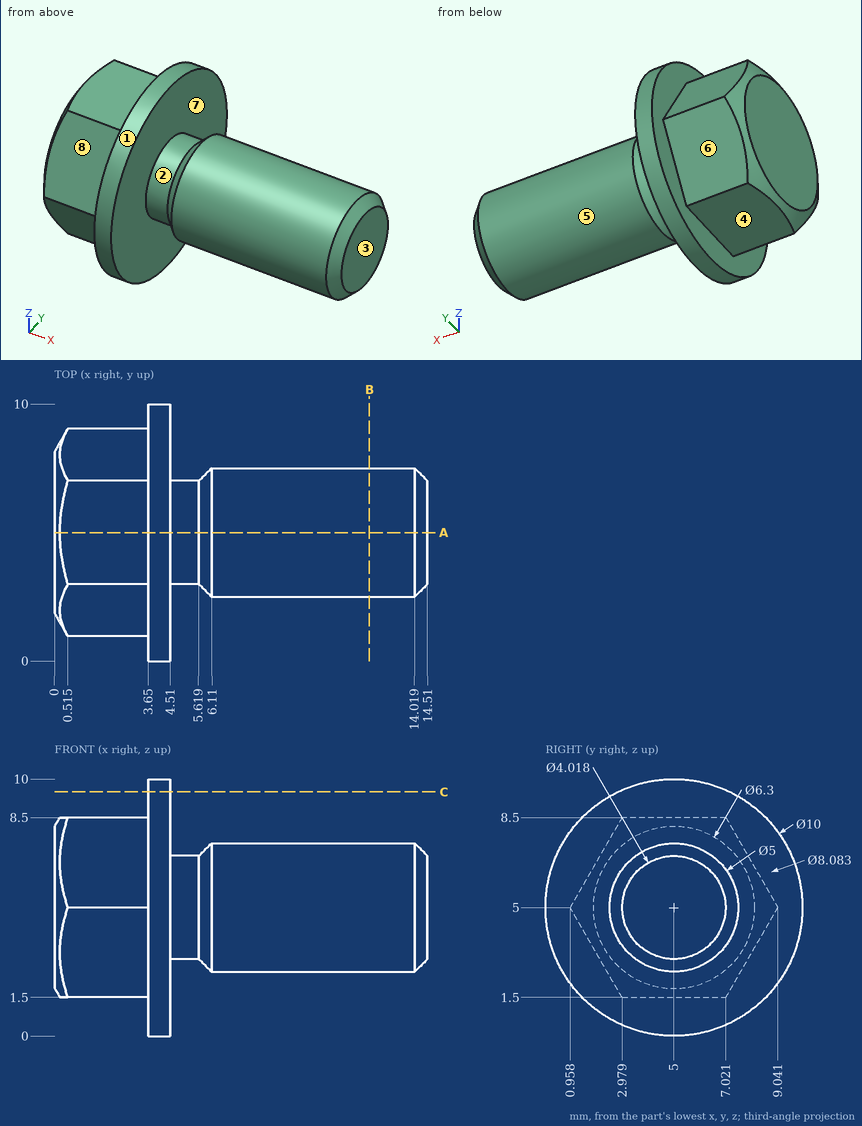
Here's the drawing with two shaded views (mm, measured from the low corner). I have some questions. A direction names the side the tool comes from. Give positions to 0.01 mm unless a question says otherwise; leave off trailing zeros. Loops run counter-clockwise (first coordinate to the right, second up) from the corner with the lowest first, then second, coordinate; pieces in that order, holes last. Notation, with made-up numbers: (-39, 73.5) -> (-6, 73.5) arc R29 ccw to (-6, 100.5) -> close; hole circle Ø10 at (64.5, 29.25). An arc over 180 degrees is marked (long way). Use one line per item in the form item = value.
1) For the marked faces 4, 5, 6, 7 and 8, which set-ups out of +Z, -Z, +X, -X, +Y, -Y let a thin tool reach every point of the face, with its end or its side?
Answers:
face_4 = -Z, -X, +Y, -Y
face_5 = +X
face_6 = -Z, -X, +Y
face_7 = none
face_8 = +Z, -X, -Y
2) We'd pull the mould along X, two halves only. Please class the marked faces 1, 2 and 3: released by +X, released by -X, zero draft, split by the parting line, or undercut.
Answers:
face_1 = zero draft
face_2 = undercut
face_3 = released by +X
3) I need wall thicknesses on line 1 along Z through (x, y) = (2, 4.25); line 2 along X through (y, z) = (2.5, 5.5); line 3 along X through (y, z) = (1.5, 3.25). Which ranges of each line are inside material? Lowest first, please.
Answers:
line_1 = 1.5 to 8.5
line_2 = 0 to 4.51
line_3 = 3.65 to 4.51
4) If we section it at B-B (x = 12.25): Please give me the cut outline in (y, z).
Answers:
outline = circle Ø5 at (5, 5)
5) If we section it at A-A (y = 5): Please give me the cut outline in (x, z).
Answers:
outline = (0, 1.85) -> (0.2, 1.5) -> (3.65, 1.5) -> (3.65, 0) -> (4.51, 0) -> (4.51, 2.99) -> (5.62, 2.99) -> (6.11, 2.5) -> (14.02, 2.5) -> (14.51, 2.99) -> (14.51, 7.01) -> (14.02, 7.5) -> (6.11, 7.5) -> (5.62, 7.01) -> (4.51, 7.01) -> (4.51, 10) -> (3.65, 10) -> (3.65, 8.5) -> (0.2, 8.5) -> (0, 8.15) -> close
6) If we section it at C-C (z = 9.5): Please give me the cut outline in (x, y).
Answers:
outline = (3.65, 2.82) -> (4.51, 2.82) -> (4.51, 7.18) -> (3.65, 7.18) -> close
7) Will these pins go through, and if not, where does the flat tip stop? pin 1 (4 mm diameter, centred on x = 1, y = 5, fed in from -Z); pin 2 (1 mm diameter, centred on x = 2.5, y = 4.5, fed in from +Z); pin 3 (4 mm diameter, centred on x = 11, y = 3, fed in from -Z).
Answers:
pin_1 = 1.5
pin_2 = 8.5
pin_3 = 2.5
